```python
from build123d import *

# Parameters (mm, degrees)
SKETCH1_R                    = 35
BOSS_EXTRUDE1_DEPTH          = 23
SKETCH2_R                    = 40
BOSS_EXTRUDE2_DEPTH          = 22
BOSS_EXTRUDE3_DEPTH          = 21
CHAMFER1_SIZE                = 0.5
CIRPATTERN1_COUNT            = 4
CHAMFER1_OF_CIRPATTERN1_SIZE = 0.5
CUT_EXTRUDE1_REACH           = 74.284
CIRPATTERN2_COUNT            = 2
CIRPATTERN2_ANGLE            = 90.0000000000002
CHAMFER2_SIZE                = 0.5


with BuildPart() as part:
    # Sketch1 → Boss-Extrude1 (new body)
    with BuildSketch(Plane.XY):
        Circle(SKETCH1_R)
    extrude(amount=BOSS_EXTRUDE1_DEPTH)

    # Sketch2 → Boss-Extrude2 (add)
    with BuildSketch(Plane.XY.offset(23)):
        Circle(SKETCH2_R)
    extrude(amount=BOSS_EXTRUDE2_DEPTH)

    # Sketch3 → Boss-Extrude3 (add)
    with BuildSketch(Plane.XY.offset(45)):
        with BuildLine():
            ThreePointArc((-4.365000000000002, 23.599719807658737), (-2.1916574340201898, 23.89972045217065), (-3.535e-13, 24.000000000000004))
            Line((0, 24.000000000000004), (0, 40))
            ThreePointArc((2.45e-15, 40), (-5.332266542853259, 39.64299349842249), (-10.569350394509378, 38.578346675798386))
            Line((-10.569350394509376, 38.578346675798386), (-4.365000000000001, 23.599719807658737))
        make_face()
        with BuildLine():
            Line((0, 40), (0, 24.000000000000004))
            ThreePointArc((-3.535e-13, 24.000000000000004), (2.1916574340198385, 23.899720452170683), (4.365000000000001, 23.599719807658737))
            Line((4.365000000000001, 23.599719807658737), (10.569350394509376, 38.578346675798386))
            ThreePointArc((10.569350394509375, 38.578346675798386), (5.332266542853264, 39.64299349842249), (2.45e-15, 40))
        make_face()
    boss_extrude3 = extrude(amount=BOSS_EXTRUDE3_DEPTH)

    # Chamfer1
    chamfer1_edges = [part.edges().sort_by_distance(p)[0] for p in [
        (-2.22e-15, 24.000000000000007, 66),
        (7.467175197254688, 31.08903324172856, 66),
        (-5.11e-15, 40.000000000000014, 66),
        (-7.467175197254688, 31.08903324172856, 66),
    ]]
    chamfer(chamfer1_edges, length=CHAMFER1_SIZE)

    # CirPattern1: Boss-Extrude3 ×4 about axis
    cirpattern1_axis = Axis((-1e-15, 7.77e-15, 0), (0, 0, 1))
    for i in range(1, CIRPATTERN1_COUNT):
        add(boss_extrude3.rotate(cirpattern1_axis, i * 360 / CIRPATTERN1_COUNT))

    # Chamfer1 of CirPattern1
    chamfer1_of_cirpattern1_edges = [part.edges().sort_by_distance(p)[0] for p in [
        (-24, 8.02e-15, 66),
        (-31.089033241728554, 7.467175197254699, 66),
        (-40.00000000000001, 6.11e-15, 66),
        (-31.089033241728554, -7.467175197254678, 66),
        (-2.72e-15, -23.999999999999993, 66),
        (-7.467175197254694, -31.089033241728547, 66),
        (-1.79e-15, -40, 66),
        (7.467175197254683, -31.089033241728547, 66),
        (24, 4.58e-15, 66),
        (31.089033241728554, -7.4671751972546865, 66),
        (40.00000000000001, 4.52e-15, 66),
        (31.089033241728554, 7.46717519725469, 66),
    ]]
    chamfer(chamfer1_of_cirpattern1_edges, length=CHAMFER1_OF_CIRPATTERN1_SIZE)

    # Sketch4 → Cut-Extrude1 (cut, up to next)
    with BuildSketch(Plane.XY.offset(45), mode=Mode.PRIVATE) as cut_extrude1_sk1:
        with BuildLine():
            Line((-4, 11.31370849898476), (-4, 15.3))
            Line((-4, 15.3), (4, 15.3))
            Line((4, 15.3), (4, 11.31370849898476))
            ThreePointArc((4, 11.31370849898476), (-2.2e-15, -11.999999999999998), (-4, 11.31370849898476))
        make_face()
    cut_extrude1_tool1 = extrude(cut_extrude1_sk1.sketch, amount=-CUT_EXTRUDE1_REACH, mode=Mode.PRIVATE) & part.part
    add(cut_extrude1_tool1.solids().sort_by_distance((0, 0.794205, 45))[0], mode=Mode.SUBTRACT)

    # Sketch6 → M8x1.25 Tapped Hole1 (revolve, cut)
    with BuildSketch(Plane(origin=(0, 0, 10), x_dir=(0, 0, 1), z_dir=(0, 1, 0))):
        Polygon((0, 0), (-9.8e-15, 40), (3.39999999999999, 40), (3.399999999999995, 3.6e-16), align=None)
    m8x1_25_tapped_hole1 = revolve(axis=Axis((-6.349999999999991, 0, 10), (1, 0, 0)), mode=Mode.SUBTRACT)

    # CirPattern2: M8x1.25 Tapped Hole1 ×2 about axis
    cirpattern2_axis = Axis((0, 0, 0), (0, 0, -1))
    for i in range(1, CIRPATTERN2_COUNT):
        add(m8x1_25_tapped_hole1.rotate(cirpattern2_axis, i * CIRPATTERN2_ANGLE / (CIRPATTERN2_COUNT - 1)), mode=Mode.SUBTRACT)

    # Chamfer2
    chamfer2_edges = [part.edges().sort_by_distance(p)[0] for p in [
        (-35, 4.29e-15, 0),
        (-40, 4.9e-15, 23),
    ]]
    chamfer(chamfer2_edges, length=CHAMFER2_SIZE)


solid = part.part
```
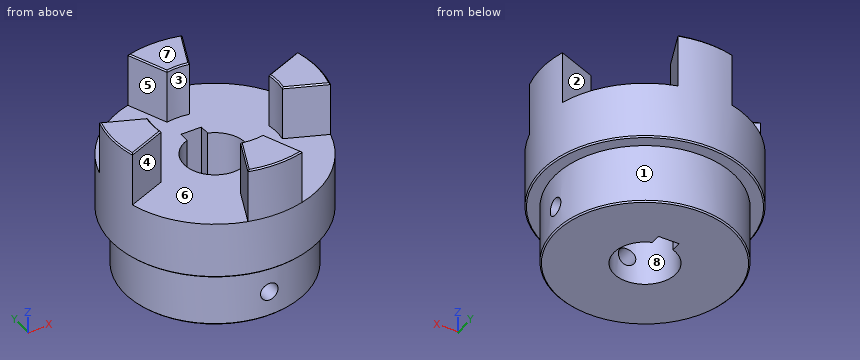
Check sheet for the modelled part. Datum: model origin and axes. Units: mm. Face numbers are marked on the shaded views. A direction names the side the tool comes from. Give positions to 0.01 mm unless a question says otherwise; leave off trailing zeros. Write each loop counter-clockwise with the first axis right and the second up, starting at its lowest first coordinate (ties: lowest second). Pieces come first, ordered by that corner, then holes.
Item 1: Cross-section at A-A (y = 0). Enter the section's corners in (x, z), and give its area (3 significant figures).
Item 2: Cross-section at B-B (x = 0). Enter the section's corners in (y, z), and give its area (3 significant figures).
Item 3: Scan lines: L1, parallel to Z at x = 26.25, y = 0; L2, parallel to Z at x = 0, y = 36.5; L3, parallel to Y at x = -1, z = 32.5. Record each from-to range of solid material in increasing order.
Item 4: Gauge pin test, flat ends, axial feed: pin 1 (19 mm diameter, centred on x = 0, y = 0, fed in from -Z); pin 2 (8 mm diameter, centred on x = -9, y = 29, fed in from +Z); pin 3 (4 mm diameter, centred on y = 0, z = 10, fed in from +X); pin 4 (2 mm diameter, centred on y = 9, z = 45.5, fed in from -X). Record the tip position at first contact, or that the pin passes through.
Item 5: Cross-section at C-C (z = 37). Enter the section's corners in (x, y), and give its area (3 significant figures).
Item 6: Draft check along X on the marked faces 5, 6, 7 and 8. Enter one of: released by +X, released by -X, zero draft, split by the parting line, or undercut.
Item 7: Access from +Z, -Z, +X, -X, +Y, -Y to the whole of each face (thin tool, end or side, straight path). Record for the marked faces 1, 2, 3 and 4.
Item 8: Cross-section at D-D (z = 12). Enter the section's corners in (x, y).
Report:
1. outline: (-40, 23.5) - (-39.5, 23) - (-35, 23) - (-35, 0.5) - (-34.5, 0) - (-12, 0) - (-12, 45) - (-24, 45) - (-24, 65.5) - (-24.5, 66) - (-39.5, 66) - (-40, 65.5) - close; (12, 0) - (34.5, 0) - (35, 0.5) - (35, 6.6) - (12, 6.6) - close; (12, 13.4) - (35, 13.4) - (35, 23) - (39.5, 23) - (40, 23.5) - (40, 65.5) - (39.5, 66) - (24.5, 66) - (24, 65.5) - (24, 45) - (12, 45) - close
1. area: 2,800 mm2
2. outline: (-40, 23.5) - (-39.5, 23) - (-35, 23) - (-35, 13.4) - (-12, 13.4) - (-12, 45) - (-24, 45) - (-24, 65.5) - (-24.5, 66) - (-39.5, 66) - (-40, 65.5) - close; (-35, 0.5) - (-34.5, 0) - (-12, 0) - (-12, 6.6) - (-35, 6.6) - close; (15.3, 0) - (34.5, 0) - (35, 0.5) - (35, 23) - (39.5, 23) - (40, 23.5) - (40, 65.5) - (39.5, 66) - (24.5, 66) - (24, 65.5) - (24, 45) - (15.3, 45) - close
2. area: 2,660 mm2
3. L1: z = 0 to 6.6, 13.4 to 66
3. L2: z = 23 to 66
3. L3: y = -39.99 to -11.96, 15.3 to 39.99
4. pin 1: passes through
4. pin 2: stops at z = 66
4. pin 3: stops at x = -11.83
4. pin 4: stops at x = -39.19
5. outline: circle Ø80 at (0, 0); hole (-4, 11.31) arc R12 ccw (long way) to (4, 11.31) - (4, 15.3) - (-4, 15.3) - close
5. area: 4,550 mm2
6. face 5: released by -X
6. face 6: undercut
6. face 7: zero draft
6. face 8: undercut
7. face 1: -Z
7. face 2: +Z, +Y
7. face 3: +Z
7. face 4: +Z, -Y
8. outline: (-4, 11.31) - (-4, 15.3) - (4, 15.3) - (4, 11.31) arc R12 cw to (11.68, 2.75) - (34.89, 2.75) arc R35 ccw (long way) to (-2.75, -34.89) - (-2.75, -11.68) arc R12 cw to start; (2.75, -34.89) arc R35 ccw to (34.89, -2.75) - (11.68, -2.75) arc R12 cw to (2.75, -11.68) - close
